from build123d import *

# Parameters (mm, degrees)
SKETCH1_W           = 180
SKETCH1_H           = 125
BOSS_EXTRUDE1_DEPTH = 100
SKETCH2_W           = 180
SKETCH2_H           = 125
BOSS_EXTRUDE2_DEPTH = 5
SKETCH3_W           = 100
SKETCH3_H           = 2.5
CUT_EXTRUDE1_DEPTH  = 200
SKETCH4_W           = 20
SKETCH4_H           = 8
BOSS_EXTRUDE4_DEPTH = 5
SKETCH5_R           = 4.5
CUT_EXTRUDE2_DEPTH  = 5


with BuildPart() as part:
    # Sketch1 → Boss-Extrude1 (new body)
    with BuildSketch(Plane(origin=(0, 0, 0), x_dir=(1, 0, 0), z_dir=(0, 1, 0))):
        Polygon((185, 5), (0, 5), (-5, 5), (-5, -130), (185, -130), align=None)
        with Locations((90, -62.5)):
            Rectangle(SKETCH1_W, SKETCH1_H, mode=Mode.SUBTRACT)
    extrude(amount=BOSS_EXTRUDE1_DEPTH)

    # Sketch2 → Boss-Extrude2 (add)
    with BuildSketch(Plane(origin=(0, 0, 0), x_dir=(-1, 0, 0), z_dir=(0, -1, 0))):
        with Locations((-90, -62.5)):
            Rectangle(SKETCH2_W, SKETCH2_H)
    extrude(amount=-BOSS_EXTRUDE2_DEPTH)

    # Sketch3 → Cut-Extrude1 (cut)
    with BuildSketch(Plane(origin=(185, 0, 0), x_dir=(0, 0, -1), z_dir=(1, 0, 0))):
        Polygon((-62.5, 10), (-52.5, 10), (-52.5, 18), (-72.5, 18), (-72.5, 10), align=None)
        Polygon((-62.5, 28), (-12.5, 28), (-12.5, 30.5), (-112.5, 30.5), (-112.5, 28), align=None)
        with Locations((-62.5, 41.75)):
            Rectangle(SKETCH3_W, SKETCH3_H)
        with Locations((-62.5, 54.25)):
            Rectangle(SKETCH3_W, SKETCH3_H)
        with Locations((-62.5, 66.75)):
            Rectangle(SKETCH3_W, SKETCH3_H)
        with Locations((-62.5, 79.25)):
            Rectangle(SKETCH3_W, SKETCH3_H)
    extrude(amount=-CUT_EXTRUDE1_DEPTH, mode=Mode.SUBTRACT)

    # Sketch4 → Boss-Extrude4 (add)
    with BuildSketch(Plane.ZY.offset(5)):
        with Locations((62.5, 14)):
            Rectangle(SKETCH4_W, SKETCH4_H)
    extrude(amount=-BOSS_EXTRUDE4_DEPTH)

    # Sketch5 → Cut-Extrude2 (cut)
    with BuildSketch(Plane.XY.offset(130)):
        with Locations((90, 50)):
            Circle(SKETCH5_R)
    extrude(amount=-CUT_EXTRUDE2_DEPTH, mode=Mode.SUBTRACT)


solid = part.part
Read the model definition and answer for the solid it produces. Units are mm, in the model's axes. A direction names the side the tool comes from. Coordinates: 2 decimals unless noted, no trailing zeros. Loops run counter-clockwise (first coordinate to the right, second up) from the corner with the lowest first, then second, coordinate; pieces in that order, holes last. Notation, with made-up numbers: (29.5, 76.25) - (68.5, 76.25) arc R22 cw to (68.5, 111.25) - close; hole circle Ø5 at (-35.5, -31.75). An arc over 180 degrees is marked (long way). Answer in a Markdown table with one row per item.
Q1. Given P1, Ø12, axis at x = 89.5, z = 19, coming from the +Y side, flat-ended and moving along its own axis, determine where the tip first touches the part or whether it passes through.
Here are the results:
| item | result |
|---|---|
| P1 | stops at y = 5 |
Q2. For faces 1 (the flat face through (-2, 40.5, 63)), 2 (the flat face through (89, 52, 0)), 3 (the flat face through (183, 18, 62)), 4 (the flat face through (-5, 51, 62)), determine the directions among +Z, -Z, +X, -X, +Y, -Y from which every point of the face is accessible in a straight line to the end or side of a thin tool.
Here are the results:
| item | result |
|---|---|
| face 1 | +X, -X |
| face 2 | +Y |
| face 3 | +X |
| face 4 | +Z, -Z, -X, +Y, -Y |
Q3. Find section D-D on z = 102.5. Count the separate pieces of the cut face and the enclosed holes in it, plus the area to 4 significant figures.
Here are the results:
| item | result |
|---|---|
| separate pieces | 11 |
| enclosed holes | 0 |
| area | 1,775 mm^2 |
Q4. Find section A-A on x = 90. Write down the section's boundary in (y, z).
Here are the results:
| item | result |
|---|---|
| outline | (0, -5) - (100, -5) - (100, 0) - (5, 0) - (5, 125) - (45.5, 125) - (45.5, 130) - (0, 130) - close; (54.5, 125) - (100, 125) - (100, 130) - (54.5, 130) - close |
Q5. Straight lines are drawn through the part: line 1 along X through (y, z) = (49, 96.5); line 2 along Z through (x, y) = (104, 82.5); line 3 along Y through (x, z) = (90, 126.1). For each, find the intervals that lie inside material, in ascending order. Write a range as [from, to].
Here are the results:
| item | result |
|---|---|
| line 1 | x = [-5, 0], [180, 185] |
| line 2 | z = [-5, 0], [125, 130] |
| line 3 | y = [0, 45.5], [54.5, 100] |
Q6. The mould has two halves that part along Z. Classify faces 5 (the flat face through (-2, 53, 63)), 6 (the cylindrical face through (86.4, 47.3, 127.5)), 7 (the flat face through (89, 38, 130)): pulls with the +Z half, pulls with the -Z half, needs draft (parallel to the pull), parting line crosses it, or undercut.
Here are the results:
| item | result |
|---|---|
| face 5 | undercut |
| face 6 | needs draft |
| face 7 | pulls with the +Z half |
Q7. Find section C-C on y = 15. Write down the section's boundary in (x, z), plus the area to 3 significant figures.
Here are the results:
| item | result |
|---|---|
| outline | (-5, -5) - (185, -5) - (185, 52.5) - (180, 52.5) - (180, 0) - (0, 0) - (0, 125) - (180, 125) - (180, 72.5) - (185, 72.5) - (185, 130) - (-5, 130) - close |
| area | 3,050 mm^2 |
Q8. Find section B-B on y = 74. Write down the section's boundary in (x, z).
Here are the results:
| item | result |
|---|---|
| outline | (-5, -5) - (185, -5) - (185, 130) - (-5, 130) - close; hole (0, 0) - (180, 0) - (180, 125) - (0, 125) - close |
